```python
from build123d import *

# Parameters (mm, degrees)
F1_DEPTH = 50.8
F2_W     = 38.1
F2_H     = 19.05
F3_DEPTH = 63.501
F5_W     = 19.05
F5_H     = 38.1
F6_DEPTH = 38.1
F7_R     = 3.175
F8_DEPTH = 69.851


with BuildPart() as f1:
    # F0 (on Front) → F1 (new body)
    with BuildSketch(Plane.XZ):
        Polygon((-25.4, 38.1), (-63.5, 38.1), (-63.5, 0), (-38.1, -25.4), (50.8, -25.4), (50.8, 0), align=None)
    extrude(amount=F1_DEPTH)

    # F2 (on face) → F3 (cut, through all)
    with BuildSketch(Plane.XY.offset(38.1)):
        with Locations((31.75, -41.275)):
            Rectangle(F2_W, F2_H)
    extrude(amount=-F3_DEPTH, mode=Mode.SUBTRACT)

    # F5 (on offset) → F6 (join)
    with BuildSketch(Plane.YZ.offset(38.1)):
        with Locations((-22.225, 25.4)):
            Rectangle(F5_W, F5_H)
    extrude(amount=-F6_DEPTH)

    # F7 (on face) → F8 (cut, through all)
    with BuildSketch(Plane.XY.offset(44.45)):
        with Locations((9.525, -22.225)):
            Circle(F7_R)
        with Locations((28.575, -22.225)):
            Circle(F7_R)
    extrude(amount=-F8_DEPTH, mode=Mode.SUBTRACT)


solid = f1.part
```
Model file for the job. Use its own axes, mm. A direction names the side the tool comes from. Round coordinates to 2 decimals unless told otherwise and drop trailing zeros. Write each loop counter-clockwise with the first axis right and the second up, starting at its lowest first coordinate (ties: lowest second). Pieces come first, ordered by that corner, then holes. Notation, with made-up numbers: (44, 52) -> (76, 52) arc R15 ccw to (76, 68) -> close; hole circle Ø7 at (23.25, 53.25). An arc over 180 degrees is marked (long way). Answer as CSV lines item,"result".
1. Mould opens along X. For faces 6 (the face through (-63.5, -25, 19)), 7 (the face through (19, -22, 44.45)), 8 (the face through (-3.7, -19.4, 27.25)) say: +X half, -X half, draft (parallel to the pull), parting line (faces both ways), or undercut.
Resolved:
face 6,"-X half"
face 7,"draft"
face 8,"undercut"
2. Drill centre lines: line 1 (X direction, y = -20.5, z = -10); line 2 (X direction, y = -24, z = -18.5); line 3 (Y direction, x = 21, z = 22). Where is each one in solid material? Low to high.
Resolved:
line 1,"-53.5 to 6.86, 12.19 to 25.91, 31.24 to 50.8"
line 2,"-45 to 6.89, 12.16 to 25.94, 31.21 to 50.8"
line 3,"-31.75 to -12.7"
3. Slice it at B-B, the plane x = 30. List the corners of the cut face in (y, z), plus the area to 3 significant figures.
Resolved:
outline,"(-31.75, -25.4) -> (-25.06, -25.4) -> (-25.06, 44.45) -> (-31.75, 44.45) -> close; (-19.39, -25.4) -> (0, -25.4) -> (0, 10.4) -> (-12.7, 10.4) -> (-12.7, 44.45) -> (-19.39, 44.45) -> close"
area,"1,390 mm²"
4. Pin check, flat tips, straight feed: pin 1 Ø1.5 at (x, z) = (30, -0.5) entering from -Y; pin 2 Ø19 at (x, z) = (24.5, 27) entering from +Y; pin 3 Ø9.5 at (y, z) = (-40, -1.5) entering from +X. Stop position of each tip, or through.
Resolved:
pin 1,"y = -31.75"
pin 2,"y = -12.7"
pin 3,"x = 12.7"
5. Tool access for faces 1 (the face through (38.1, -22, 26)), 2 (the face through (0, -22, 35)), 3 (the face through (12.7, -41, -3)), 4 (the face through (-44, -25, 38.1)), 5 (the face through (19, -12.7, 29)): list every direction of +Z, -Z, +X, -X, +Y, -Y with a clear straight run to the whole face (end or side of a thin tool).
Resolved:
face 1,"+Z, +X, +Y, -Y"
face 2,"+Z, +Y, -Y"
face 3,"+Z, -Z, +X, -Y"
face 4,"+Z, -X, +Y, -Y"
face 5,"+Z, +X, +Y"
6. Slice it at A-A, the plane z = 29. List the corners of the cut face in (x, y) (3 decimals).
Resolved:
outline,"(-63.5, -50.8) -> (-7.2, -50.8) -> (-7.2, 0) -> (-63.5, 0) -> close; (0, -31.75) -> (38.1, -31.75) -> (38.1, -12.7) -> (0, -12.7) -> close; hole circle Ø6.35 at (9.525, -22.225); hole circle Ø6.35 at (28.575, -22.225)"
7. Slice it at D-D, the plane z = -15. List the corners of the cut face in (x, y) (3 decimals).
Resolved:
outline,"(-48.5, -50.8) -> (12.7, -50.8) -> (12.7, -31.75) -> (50.8, -31.75) -> (50.8, 0) -> (-48.5, 0) -> close; hole circle Ø6.35 at (9.525, -22.225); hole circle Ø6.35 at (28.575, -22.225)"
8. Slice it at C-C, the plane y = -47. List the corners of the cut face in (x, z), plus the area to 3 significant figures.
Resolved:
outline,"(-63.5, 0) -> (-38.1, -25.4) -> (12.7, -25.4) -> (12.7, 19.05) -> (-25.4, 38.1) -> (-63.5, 38.1) -> close"
area,"4,150 mm²"
